The drawing under review shows one solid part. Ordinate dimensions are in mm from its lowest x, y, z. A direction names the side the tool comes from. Coordinates: 2 decimals unless noted, no trailing zeros. Write each loop counter-clockwise with the first axis right and the second up, starting at its lowest first coordinate (ties: lowest second). Pieces come first, ordered by that corner, then holes. Notation, with made-up numbers: (18.5, 82.5) - (61.5, 82.5) arc R23 ccw to (61.5, 91.5) - close; hole circle Ø2 at (37, 58). An arc over 180 degrees is marked (long way). Put each result on its own line as item: value. Start each with the question number.
Item 1: Consider section C-C on y = 11.5. State how many separate pieces and enclosed holes the cut face has, then the cut area to 3 significant figures.
Item 2: Machinability: for the marked faces 4, 5 and 6, which of the approach directions +Z, -Z, +X, -X, +Y, -Y give a long, thin tool a straight path to every point of the face, cutting with its end or side? Answer none if there is none.
Item 3: Mouldability with a two-part tool opening along Z and no side actions: class the marked faces 1, 2 and 3 as pulls with the +Z half, pulls with the -Z half, needs draft (parallel to the pull), parting line crosses it, or undercut.
Item 4: Consider section B-B on x = 25. Give the boundary of the cut face in (y, z), then the cut area to 3 significant figures.
Item 5: Consider section A-A on z = 25. Give the boundary of the cut face in (x, y).
Item 6: For pin 1 (1.5 mm diameter, centred on x = 10, y = 11.5, fed in from +Z); pin 2 (1.8 mm diameter, centred on x = 25, y = 5, fed in from +Z); pin 3 (2 mm diameter, centred on x = 15, z = 13, fed in from -Y), all flat-tipped, find the tip position at first contact; note any pin that passes through.
Item 7: Consider section D-D on x = 6.25. Give the boundary of the cut face in (y, z).
Item 8: To check wall thickness, follow L1, parallel to Z at x = 25.5, y = 11 (1 decimal); L2, parallel to X at y = 8.25, z = 25; L3, parallel to Y at x = 31, z = 46. State the ranges of each line that lie inside material, in increasing order. Write a range as [from, to].
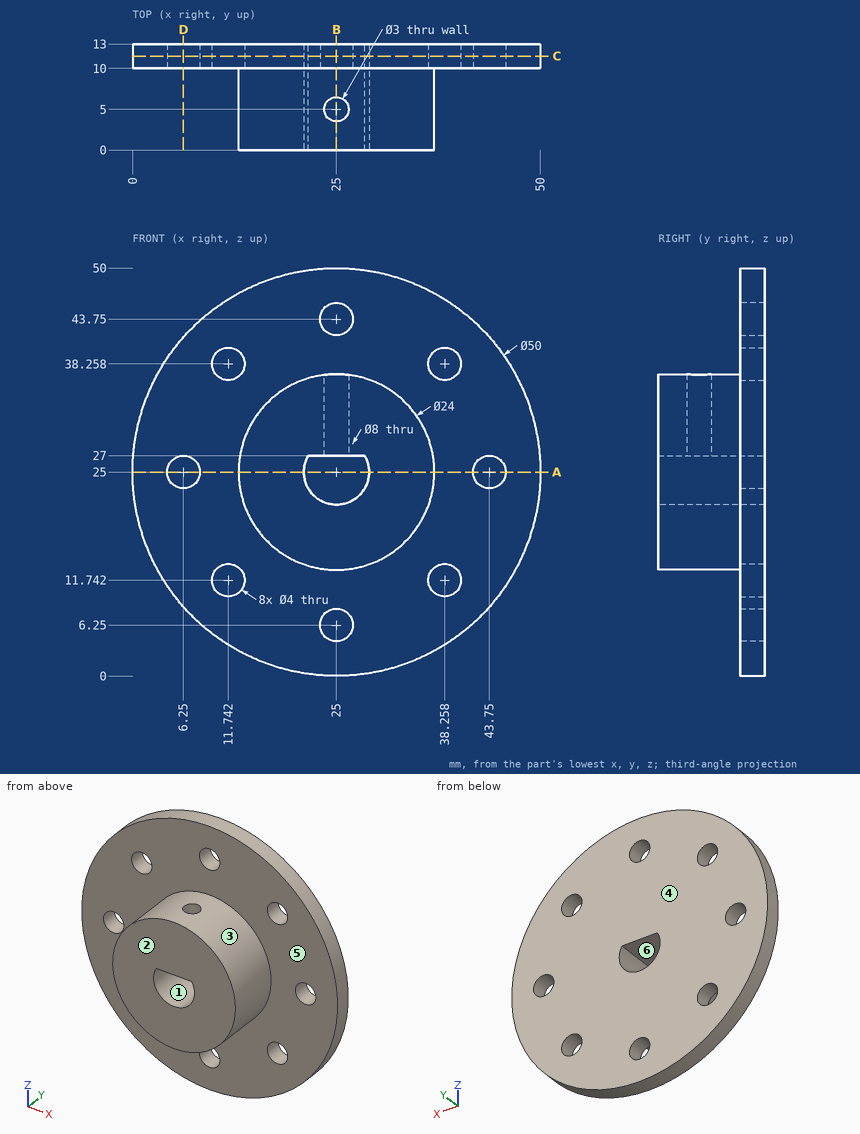
Report:
1. separate pieces: 1
1. enclosed holes: 9
1. area: 1,820 mm²
2. face 4: +Z, -Z, +X, -X, +Y
2. face 5: -Y
2. face 6: +Y, -Y
3. face 1: undercut
3. face 2: needs draft
3. face 3: parting line crosses it
4. outline: (0, 13) - (10, 13) - (10, 8.25) - (13, 8.25) - (13, 21) - (0, 21) - close; (0, 27) - (3.5, 27) - (3.5, 37) - (0, 37) - close; (6.5, 27) - (13, 27) - (13, 41.75) - (10, 41.75) - (10, 37) - (6.5, 37) - close; (10, 0) - (13, 0) - (13, 4.25) - (10, 4.25) - close; (10, 45.75) - (13, 45.75) - (13, 50) - (10, 50) - close
4. area: 258 mm²
5. outline: (0, 10) - (4.25, 10) - (4.25, 13) - (0, 13) - close; (8.25, 10) - (13, 10) - (13, 0) - (21, 0) - (21, 13) - (8.25, 13) - close; (29, 0) - (37, 0) - (37, 10) - (41.75, 10) - (41.75, 13) - (29, 13) - close; (45.75, 10) - (50, 10) - (50, 13) - (45.75, 13) - close
6. pin 1: z = 45.54
6. pin 2: z = 21.1
6. pin 3: y = 10
7. outline: (10, 8.46) - (13, 8.46) - (13, 23) - (10, 23) - close; (10, 27) - (13, 27) - (13, 41.54) - (10, 41.54) - close
8. L1: [0, 4.3], [8.2, 21], [27, 41.8], [45.7, 50]
8. L2: [13, 21], [29, 37]
8. L3: [10, 13]
